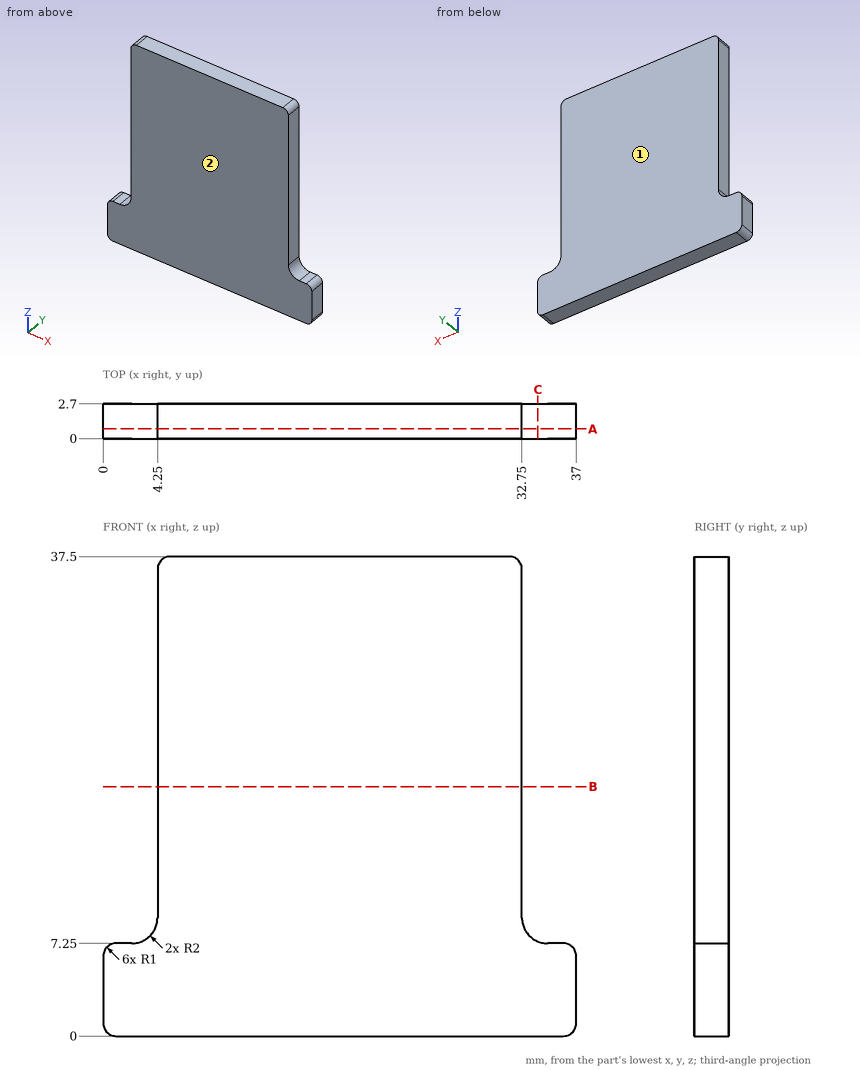
Source: three-view drawing plus pictorial views. Frame: mm from the lowest corner of the part. Round coordinates to 2 decimals unless told otherwise and drop trailing zeros. Loops run counter-clockwise (first coordinate to the right, second up) from the corner with the lowest first, then second, coordinate; pieces in that order, holes last. Notation, with made-up numbers: M 63.25,-2 L 106.25,-2 A26 ccw 106.25,14 Z; hole C -8.5,70 d9. An arc over 180 degrees is marked long. Put each result on its own line as item: value. Start each with the question number.
(1) Section query C-C (x = 34). Return loops of the section in (y, z), then the cut area to 3 significant figures.
(2) Section query A-A (y = 0.75). Return loops of the section in (x, z), then the cut area to 3 significant figures.
(3) Contact query for flat-ended pins moving along their axis: pin 1 Ø1.4 at (x, y) = (35.5, 1) entering from +Z; pin 2 Ø1 at (y, z) = (2, 24.5) entering from -X; pin 3 Ø1 at (x, z) = (13.5, 27) entering from -Y. Output: stop coordinate, or through.
(4) Draft query along Y for the marked faces 1 and 2. Return one class per face: +Y half, -Y half, draft (parallel to the pull), parting line (faces both ways), or undercut.
(5) Material intervals for line 1 along X through (y, z) = (2.5, 21.5); line 2 along Z through (x, y) = (2, 1.6); line 3 along Z through (x, y) = (33, 0.3), sorted ascending. Write a range as [from, to].
(6) Section query B-B (z = 19.5). Return loops of the section in (x, y), then the cut area to 4 significant figures.
Findings below:
1. outline: M 0,0 L 2.7,0 L 2.7,7.4 L 0,7.4 Z
1. area: 20.0 mm2
2. outline: M 0,1 A1 ccw 1,0 L 36,0 A1 ccw 37,1 L 37,6.25 A1 ccw 36,7.25 L 34.75,7.25 A2 cw 32.75,9.25 L 32.75,36.5 A1 ccw 31.75,37.5 L 5.25,37.5 A1 ccw 4.25,36.5 L 4.25,9.25 A2 cw 2.25,7.25 L 1,7.25 A1 ccw 0,6.25 Z
2. area: 1,130 mm2
3. pin 1: stops at z = 7.25
3. pin 2: stops at x = 4.25
3. pin 3: stops at y = 0
4. face 1: +Y half
4. face 2: -Y half
5. line 1: x = [4.25, 32.75]
5. line 2: z = [0, 7.25]
5. line 3: z = [0, 8.28]
6. outline: M 4.25,0 L 32.75,0 L 32.75,2.7 L 4.25,2.7 Z
6. area: 76.95 mm2
